```python
from build123d import *

# Parameters (mm, degrees)
BOSS_EXTRUDE2_DEPTH = 3.175
CHAMFER3_SIZE       = 2.6


with BuildPart() as part:
    # Sketch2 → Boss-Extrude2 (new body)
    with BuildSketch(Plane.XY):
        Polygon((33.967630838, -35.823456397), (25.63439182, 59.425901431), (0, 64.888689731), (-25.63439182, 59.425901431), (-33.967630838, -35.823456397), (0, -64.691310269), align=None)
        Polygon((-30.464841537, 4.213608519), (-28.721726682, 24.137502481), (-32.407647065, 24.459978729), (-34.15076192, 4.536084767), align=None)
        Polygon((32.407647065, 24.459978729), (28.721726682, 24.137502481), (30.464841537, 4.213608519), (34.15076192, 4.536084767), align=None)
        Polygon((27.2046006, -46.164342336), (24.938042288, -43.497375254), (9.698230388, -56.449137036), (11.9647887, -59.116104119), align=None)
        Polygon((-9.698230388, -56.449137036), (-24.938042288, -43.497375254), (-27.2046006, -46.164342336), (-11.9647887, -59.116104119), align=None)
    extrude(amount=BOSS_EXTRUDE2_DEPTH)

    # Chamfer3
    chamfer3_edges = [part.edges().sort_by_distance(p)[0] for p in [
        (19.58469465, -52.640223227, 3.175),
        (33.279204493, 14.498031748, 3.175),
        (-33.279204493, 14.498031748, 3.175),
        (-19.58469465, -52.640223227, 3.175),
    ]]
    chamfer(chamfer3_edges, length=CHAMFER3_SIZE)


solid = part.part
```
Could you check a few things on this model? Use its own coordinates, in mm. A direction names the side the tool comes from. Coordinates: 2 decimals unless noted, no trailing zeros. Loops run counter-clockwise (first coordinate to the right, second up) from the corner with the lowest first, then second, coordinate; pieces in that order, holes last. Notation, with made-up numbers: M -11,-21 L 37,-21 A24 ccw 37,5 Z; hole C -39.5,58 d3. An arc over 180 degrees is marked long. Put each result on its own line as item: value. Start each with the question number.
(1) For faces 1 (the face through (-12.638, 62.196, 1.565)), 2 (the face through (4.78, -60.63, 1.57)), 3 (the face through (31.872, 4.337, 1.212)), 4 (the face through (19.48, -52.73, 0.28)), 5 (the face through (-29.516, -39.607, 1.565)), which set-ups out of +Z, -Z, +X, -X, +Y, -Y let a thin tool reach every point of the face, with its end or its side?
(2) Suppose I cut it at C-C on y = 19. Please give me the cut outline in (x, z) (3 decimals), then the cut area to 3 significant figures.
(3) Suppose I cut it at A-A on z = 1.8. Please give me the cut outline in (x, y), then the cut area to 3 significant figures.
(4) I need wall thicknesses on line 1 (X direction, y = -19, z = 0.9); line 2 (Y direction, x = -29.5, z = 1.6); line 3 (X direction, y = 32, z = 0.1). Which ranges of each line are inside material? Lowest first, please. Write a range as from..to.
(5) Suppose I cut it at B-B on x = -13.5. Please give me the cut outline in (y, z) (3 decimals), then the cut area to 3 significant figures.
(6) Thinking about a two-plate mould opening in X: for faces 6 (the face through (10.564, -57.468, 1.212)), 7 (the face through (-31.92, 4.34, 1.21)), 8 (the face through (30.181, 24.265, 1.212)), 9 (the face through (0, 1, 0)), which applies, pulls with the +X half, pulls with the -X half, needs draft (parallel to the pull), parting line crosses it, or undercut?
(7) Suppose I cut it at D-D on x = -22.5. Please give me the cut outline in (y, z) (1 decimal).
Solutions:
1. face 1: +Z, -Z, -X, +Y
1. face 2: +Z, -Z, -Y
1. face 3: +Z, -Z, +X
1. face 4: +Z, -Z, +X, -Y
1. face 5: +Z, -Z, -X
2. outline: M -32.885,0 L 32.885,0 L 32.885,0.575 L 30.275,3.175 L -30.275,3.175 L -32.885,0.575 Z
2. area: 202 mm2
3. outline: M -33.97,-35.82 L -24.94,-43.5 L -26.41,-45.23 L -11.17,-58.18 L -9.7,-56.45 L 0,-64.69 L 9.7,-56.45 L 11.17,-58.18 L 26.41,-45.23 L 24.94,-43.5 L 33.97,-35.82 L 30.46,4.21 L 32.93,4.43 L 31.19,24.35 L 28.72,24.14 L 25.63,59.43 L 0,64.89 L -25.63,59.43 L -28.72,24.14 L -31.19,24.35 L -32.93,4.43 L -30.46,4.21 Z
3. area: 6,990 mm2
4. line 1: x = -32.5..32.5
4. line 2: y = -39.62..24.21
4. line 3: x = -28.03..28.03
5. outline: M -57.811,0 L 62.012,0 L 62.012,3.175 L -54.399,3.175 L -57.811,0.575 Z
5. area: 376 mm2
6. face 6: undercut
6. face 7: pulls with the -X half
6. face 8: undercut
6. face 9: needs draft
7. outline: M -50.2,0 L 60.1,0 L 60.1,3.2 L -46.8,3.2 L -50.2,0.6 Z
